Could you check a few things on this drawing? It's one solid part, dimensions in mm from its lowest x, y, z. A direction names the side the tool comes from. Round coordinates to 2 decimals unless told otherwise and drop trailing zeros. Loops run counter-clockwise (first coordinate to the right, second up) from the corner with the lowest first, then second, coordinate; pieces in that order, holes last. Notation, with made-up numbers: (17, 31.5) -> (25, 31.5) arc R26 ccw to (25, 66.5) -> close; hole circle Ø6 at (-11, -39). An arc over 180 degrees is marked (long way). Use one line per item in the form item = value. Start each with the question number.
Item 1: If we section it at A-A (x = 46.5): Write out the boundary of the cut face in (y, z).
Item 2: I'm going to push flat-ended pins straight in: pin 1 Ø0.6 at (x, y) = (35, 2.5) entering from +Z; pin 2 Ø1.6 at (x, y) = (23, 2.5) entering from -Z; pin 3 Ø4 at (x, z) = (38.5, 11) entering from -Y; pin 4 Ø1 at (y, z) = (3, 7.5) entering from +X. Where does each tip first touch, or does it pass through?
Item 3: For the marked faces 1 and 2, which set-ups out of +Z, -Z, +X, -X, +Y, -Y let a thin tool reach every point of the face, with its end or its side?
Item 4: If we section it at C-C (y = 0.9): Write out the boundary of the cut face in (x, z).
Item 5: If we section it at D-D (z = 6.5): Write out the boundary of the cut face in (x, y), then the cut area to 3 significant figures.
Item 6: If we section it at B-B (z = 11.5): Write out the boundary of the cut face in (x, y).
Item 7: If I drill on L1, parallel to X at y = 0.7, z = 9.5; L2, parallel to X at y = 2.3, z = 10.5; L3, parallel to Z at x = 39, y = 2.2, over which ranges is the centre line in solid material (lowest first)? Write a range as [from, to].
Item 8: Thinking about a two-plate mould opening in X: for the marked faces 3 and 4, which applies, released by +X, released by -X, zero draft, split by the parting line, or undercut?
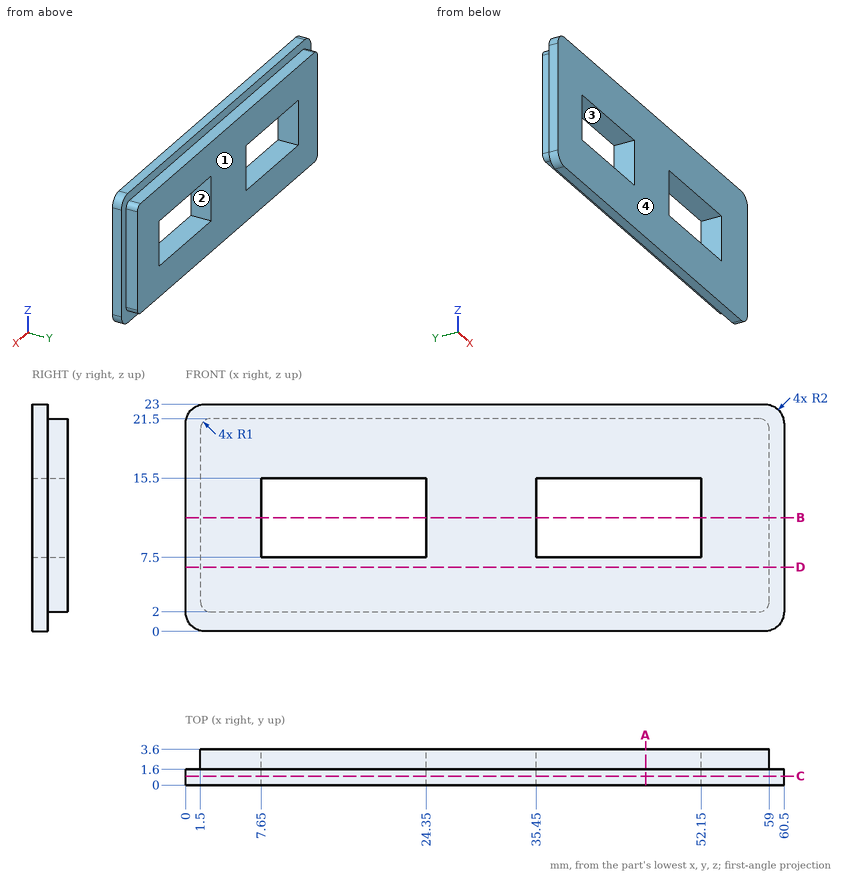
Values found:
q1.outline = (0, 0) -> (1.6, 0) -> (1.6, 2) -> (3.6, 2) -> (3.6, 7.5) -> (0, 7.5) -> close; (0, 15.5) -> (3.6, 15.5) -> (3.6, 21.5) -> (1.6, 21.5) -> (1.6, 23) -> (0, 23) -> close
q2.pin_1 = 21.5
q2.pin_2 = 2
q2.pin_3 = through
q2.pin_4 = 59
q3.face_1 = +Z, -Z, +X, -X, +Y
q3.face_2 = +Y, -Y
q4.outline = (0, 2) arc R2 ccw to (2, 0) -> (58.5, 0) arc R2 ccw to (60.5, 2) -> (60.5, 21) arc R2 ccw to (58.5, 23) -> (2, 23) arc R2 ccw to (0, 21) -> close; hole (7.65, 7.5) -> (24.35, 7.5) -> (24.35, 15.5) -> (7.65, 15.5) -> close; hole (35.45, 7.5) -> (52.15, 7.5) -> (52.15, 15.5) -> (35.45, 15.5) -> close
q5.outline = (0, 0) -> (60.5, 0) -> (60.5, 1.6) -> (59, 1.6) -> (59, 3.6) -> (1.5, 3.6) -> (1.5, 1.6) -> (0, 1.6) -> close
q5.area = 212 mm2
q6.outline = (0, 0) -> (7.65, 0) -> (7.65, 3.6) -> (1.5, 3.6) -> (1.5, 1.6) -> (0, 1.6) -> close; (24.35, 0) -> (35.45, 0) -> (35.45, 3.6) -> (24.35, 3.6) -> close; (52.15, 0) -> (60.5, 0) -> (60.5, 1.6) -> (59, 1.6) -> (59, 3.6) -> (52.15, 3.6) -> close
q7.L1 = [0, 7.65], [24.35, 35.45], [52.15, 60.5]
q7.L2 = [1.5, 7.65], [24.35, 35.45], [52.15, 59]
q7.L3 = [2, 7.5], [15.5, 21.5]
q8.face_3 = undercut
q8.face_4 = zero draft
